The model under review builds one solid part; all positions refer to its coordinate system, in mm. A direction names the side the tool comes from. Round coordinates to 2 decimals unless told otherwise and drop trailing zeros. Order: outer loops, then holes, each group sorted by start corner. A loop starts at its lowest first (then second) coordinate and runs counter-clockwise, first axis right, second up.
Autodesk Inventor part; units mm, degrees
ref_plane "YZ Plane" through (0, 0, 0) normal (1, 0, 0) x (0, 1, 0)
ref_plane "XZ Plane" through (0, 0, 0) normal (0, 1, 0) x (-1, 0, 0)
ref_plane "XY Plane" through (0, 0, 0) normal (0, 0, 1) x (1, 0, 0)
sketch "Sketch1" plane through (0, 0, 0) normal (0, 0, 1) x (1, 0, 0)
  line L0 (0, 0) -> (10, 0)
  circle A0 centre (0, 0) radius 1.5
  circle A1 centre (10, 0) radius 1.5
  circle A2 centre (0, 0) radius 2.5
  circle A3 centre (10, 0) radius 2.5
  line L1 (0, -2.5) -> (10, -2.5)
  line L2 (-2.5, 0) -> (-2.5, 5)
  line L3 (-2.5, 5) -> (0, 19.1782)
  line L4 (-2.5, 5) -> (11.8969, 5) construction
  line L5 (0, 19.1782) -> (0, 29.1782)
  line L6 (0, 29.1782) -> (0.8682, 34.1022)
  line L7 (0.8682, 34.1022) -> (5.8682, 34.1022)
  line L8 (5.8682, 34.1022) -> (5.8682, 29.1022)
  line L9 (5.8682, 29.1022) -> (4.8422, 26.2832)
  line L10 (4.8422, 26.2832) -> (4.3644, 10.2903)
  line L11 (4.3644, 10.2903) -> (12.5, 7.0509)
  line L12 (12.5, 7.0509) -> (12.5, 0)
  line L13 (5.8682, 34.1022) -> (14.2847, 34.1022)
  line L14 (14.2847, 34.1022) -> (14.2847, 29.1022)
  line L15 (14.2847, 29.1022) -> (5.8682, 29.1022)
  dimension "d0" = 10
  dimension "d1" = 3
  dimension "d2" = 3
  dimension "d3" = 5
  dimension "d4" = 5
  dimension "d5" = 5
  dimension "d6" = 80
  dimension "d7" = 10
  dimension "d8" = 5
  dimension "d9" = 170
  dimension "d10" = 5
  dimension "d11" = 5
  dimension "d12" = 3
  dimension "d13" = 160
  dimension "d14" = 16
  dimension "d15" = 110
extrude "Extrusion1" add sketch "Sketch1" along normal blind 5 contours A2 | A2 L2 L3 L5 L6 L7 L8 L9 L10 L11 L12 A3 L0 | L0 A3 L1 A2 | A3
sketch "Sketch2" plane through (0, 0, 0) normal (0, 0, -1) x (-1, 0, 0)
  line L0 (-5.8682, 34.1022) -> (-0.8682, 34.1022)
  line L1 (-0.8682, 34.1022) -> (-13.6111, 34.1022)
  line L2 (-13.6111, 34.1022) -> (-13.6111, 29.3872)
  line L3 (-13.6111, 29.3872) -> (-0.8682, 29.3872)
  line L4 (-0.8682, 29.3872) -> (-0.8682, 34.1022)
  point P0 (0, 0)
extrude "Extrusion3" add sketch "Sketch2" along normal blind 2
properties part number "gripper"
(1) Draft analysis for pull direction X (two halves, no side actions). For faces 6 (the cylindrical face through (-1.5, -0.07, 2.46)), 7 (the flat face through (3, 8, 0)), 8 (the flat face through (5.36, 27.71, 2.46)), state which applies: pulls with the +X half, pulls with the -X half, needs draft (parallel to the pull), parting line crosses it, or undercut.
Data:
face 6: undercut
face 7: needs draft
face 8: pulls with the +X half
(2) Insertion check: pin 1 (4.5 mm diameter, centred on x = 5.5, y = 16, fed in from -Z); pin 2 (1.8 mm diameter, centred on x = 0, y = 0, fed in from +Z); pin 3 (3.5 mm diameter, centred on x = 10, y = 0, fed in from +Z); pin 4 (3 mm diameter, centred on y = 25, z = 1.5, fed in from -X). Each pin has a flat end and moves straight along its axis. Give the tip position at first contact, or say it passes through.
Data:
pin 1: stops at z = 0
pin 2: passes through
pin 3: stops at z = 5
pin 4: stops at x = 0
(3) To check wall thickness, follow probe 1 along X at (y, z) = (-0.5, 2.25); probe 2 along Z at (x, y) = (1.5, 17); probe 3 along Y at (x, z) = (11.75, -0.5). State the ranges of each line that lie inside material, in increasing order.
Data:
probe 1: x = -2.45 to -1.41, 1.41 to 8.59, 11.41 to 12.45
probe 2: z = 0 to 5
probe 3: y = 29.39 to 34.1
(4) For faces 1 (the flat face through (10, 32, 0)), 2 (the flat face through (0.868, 32, -1)), 3 (the flat face through (8.38, 8.69, 2.46)), 4 (the flat face through (0, 24, 2)), 5 (the flat face through (7, 29.387, -1)), list the 3-axis set-ups (+Z, -Z, +X, -X, +Y, -Y) from which the entire face can be reached by the end or side of a thin tool; tool diameter is ignored.
Data:
face 1: +Z, +X, +Y
face 2: -Z, -X, +Y, -Y
face 3: +Z, -Z, +X
face 4: +Z, -Z, -X, +Y
face 5: -Z, +X, -X, -Y
(5) Consider section D-D (y = 25.5). Write out the cut boundary in (x, z).
Data:
outline: (0, 0) - (4.82, 0) - (4.82, 5) - (0, 5) - close
(6) Consider section C-C (z = -1). Write out the cut boundary in (x, y).
Data:
outline: (0.87, 29.39) - (13.61, 29.39) - (13.61, 34.1) - (0.87, 34.1) - close
(7) Consider section B-B (x = 9). Write out the cut boundary in (y, z).
Data:
outline: (-2.5, 0) - (-1.12, 0) - (-1.12, 5) - (-2.5, 5) - close; (1.12, 0) - (8.44, 0) - (8.44, 5) - (1.12, 5) - close; (29.39, -2) - (34.1, -2) - (34.1, 0) - (29.39, 0) - close
(8) Consider section A-A (z = 2). Write out the cut boundary in (x, y).
Data:
outline: (-2.5, 0) arc R2.5 ccw to (0, -2.5) - (10, -2.5) arc R2.5 ccw to (12.5, 0) - (12.5, 7.05) - (4.36, 10.29) - (4.84, 26.28) - (5.87, 29.1) - (5.87, 34.1) - (0.87, 34.1) - (0, 29.18) - (0, 19.18) - (-2.5, 5) - close; hole circle Ø3 at (0, 0); hole circle Ø3 at (10, 0)
